Could you check a few things on this model? Use its own coordinates, in mm. A direction names the side the tool comes from. Give positions to 0.01 mm unless a question says otherwise; leave off trailing zeros. Loops run counter-clockwise (first coordinate to the right, second up) from the corner with the lowest first, then second, coordinate; pieces in that order, holes last. Notation, with made-up numbers: (29, 23) -> (55, 23) arc R30 cw to (55, 51) -> close; hole circle Ø4 at (68.25, -4.75). An arc over 180 degrees is marked (long way). Write item = value, one per line. Start each with the question number.
1) I want a section at A-A (z = 29). List the corners of the cut face in (x, y) for me.
2) On a 3-axis mill with a long thin cutter (end or side, diameter ignored), from which of +Z, -Z, +X, -X, +Y, -Y can I reach the whole of each face in a straight line? I mean faces 4 (the face through (2, -13.354, 20)), 5 (the face through (-5, 21.646, 19)), 6 (the face through (3.753, 26.484, 2.028)), 7 (the face through (5, -7.354, 20)). Say none if no direction works.
3) I'm going to push flat-ended pins straight in: pin 1 Ø10 at (x, z) = (-2, 14.5) entering from -Y; pin 2 Ø1.5 at (x, y) = (7, -14) entering from -Z; pin 3 Ø3.5 at (x, z) = (4.87, 22) entering from +Y; pin 4 Ø2 at (x, z) = (-5.5, 16) entering from +Y. Where does each tip first touch, or does it pass through?
4) If we mould it in two halves opening along Z, with no side actions, what happens to faces 1 (the face through (4.674, -10.396, 23.487)), 2 (the face through (2, -24, 4)), 3 (the face through (-2.631, 7, 19))? For each: +Z half, -Z half, draft (parallel to the pull), parting line (faces both ways), or undercut.
5) I want a section at D-D (x = 2.25). List the corners of the cut face in (y, z) for me, and give its area (3 significant figures).
6) I want a section at B-B (x = 7.75). List the corners of the cut face in (y, z) for me, and give its area (3 significant figures).
7) I need wall thicknesses on probe 1 along Y at (x, z) = (3.5, 6); probe 2 along X at (y, z) = (14.5, 28.5); probe 3 along Z at (x, y) = (9.75, 12.5). Which ranges of each line are inside material? Lowest first, please. Write a range as from..to.
8) I want a section at C-C (y = 5.5). List the corners of the cut face in (x, z) for me, and give its area (3 significant figures).
from build123d import *

# Parameters (mm, degrees)
BOSS_EXTRUDE1_DEPTH = 35
SKETCH3_R           = 1.5
CUT_EXTRUDE1_DEPTH  = 15
LPATTERN1_COUNT     = 3
LPATTERN1_PITCH     = 7
SKETCH6_W           = 15
SKETCH6_H           = 35
SKETCH6_R           = 1.5
BOSS_EXTRUDE4_DEPTH = 6
SKETCH7_W           = 15
SKETCH7_H           = 35
CUT_EXTRUDE2_DEPTH  = 8
SKETCH2_W           = 4
SKETCH2_H           = 35
BOSS_EXTRUDE5_DEPTH = 20
BOSS_EXTRUDE6_DEPTH = 15
SKETCH10_W          = 20
SKETCH10_H          = 4
BOSS_EXTRUDE7_DEPTH = 15
SKETCH11_R          = 3
CUT_EXTRUDE3_DEPTH  = 15


with BuildPart() as part:
    # Sketch1 → Boss-Extrude1 (new body)
    with BuildSketch(Plane.XY):
        Polygon((12.368951074, 15.64566438), (-2.631048926, 15.64566438), (-2.631048926, -13.35433562), (-7.631048926, -13.35433562), (-7.631048926, 21.64566438), (12.368951074, 21.64566438), align=None)
    extrude(amount=BOSS_EXTRUDE1_DEPTH)

    # Sketch3 → Cut-Extrude1 (cut)
    with BuildSketch(Plane.XZ.offset(-15.64566438)):
        with Locations((4.868951074, 29)):
            Circle(SKETCH3_R)
    cut_extrude1 = extrude(amount=-CUT_EXTRUDE1_DEPTH, mode=Mode.SUBTRACT)

    # LPattern1: Cut-Extrude1 ×3
    with Locations(*[(0, 0, -i * LPATTERN1_PITCH) for i in range(1, LPATTERN1_COUNT)]):
        add(cut_extrude1, mode=Mode.SUBTRACT)

    # Sketch6 → Boss-Extrude4 (add)
    with BuildSketch(Plane.XZ.offset(13.35433562)):
        with Locations((4.868951074, 17.5)):
            Rectangle(SKETCH6_W, SKETCH6_H)
        with Locations((4.868951074, 15)):
            Circle(SKETCH6_R, mode=Mode.SUBTRACT)
        with Locations((4.868951074, 29)):
            Circle(SKETCH6_R, mode=Mode.SUBTRACT)
        with Locations((4.868951074, 22)):
            Circle(SKETCH6_R, mode=Mode.SUBTRACT)
    extrude(amount=-BOSS_EXTRUDE4_DEPTH)

    # Sketch7 → Cut-Extrude2 (cut)
    with BuildSketch(Plane.XZ.offset(-15.64566438)):
        with Locations((4.868951074, 17.5)):
            Rectangle(SKETCH7_W, SKETCH7_H)
    extrude(amount=-CUT_EXTRUDE2_DEPTH, mode=Mode.SUBTRACT)

    # Sketch2 → Boss-Extrude5 (add)
    with BuildSketch(Plane.ZY.offset(7.631048926)):
        with Locations((2, 4.14566438)):
            Rectangle(SKETCH2_W, SKETCH2_H)
    extrude(amount=-BOSS_EXTRUDE5_DEPTH)

    # Sketch9 → Boss-Extrude6 (add)
    with BuildSketch(Plane(origin=(0, 21.64566438, 0), x_dir=(1, 0, 0), z_dir=(0, 1, 0))):
        Polygon((-2.631048926, -4), (-7.631048926, -4), (-7.631048926, 0), (12.368951074, 0), (12.368951074, -4), align=None)
    extrude(amount=BOSS_EXTRUDE6_DEPTH)

    # Sketch10 → Boss-Extrude7 (add)
    with BuildSketch(Plane.XZ.offset(13.35433562)):
        with Locations((2.368951074, 2)):
            Rectangle(SKETCH10_W, SKETCH10_H)
    extrude(amount=BOSS_EXTRUDE7_DEPTH)

    # Sketch11 → Cut-Extrude3 (cut)
    with BuildSketch(Plane.XY.offset(4)):
        with Locations((2.368951074, -20.85433562)):
            Circle(SKETCH11_R)
        with Locations((2.368951074, 29.14566438)):
            Circle(SKETCH11_R)
    extrude(amount=-CUT_EXTRUDE3_DEPTH, mode=Mode.SUBTRACT)


solid = part.part
Answer list:
q1.outline = (-7.63, -13.35) -> (3.37, -13.35) -> (3.37, -7.35) -> (-2.63, -7.35) -> (-2.63, 21.65) -> (-7.63, 21.65) -> close; (6.37, -13.35) -> (12.37, -13.35) -> (12.37, -7.35) -> (6.37, -7.35) -> close
q2.face_4 = +Z, +X, -X, -Y
q2.face_5 = +Z, +X, -X, +Y
q2.face_6 = +Z, -Z
q2.face_7 = +Z, +X, +Y
q3.pin_1 = -13.35
q3.pin_2 = 0
q3.pin_3 = -7.35
q3.pin_4 = 21.65
q4.face_1 = undercut
q4.face_2 = +Z half
q4.face_3 = draft
q5.outline = (-28.35, 0) -> (-23.85, 0) -> (-23.85, 4) -> (-28.35, 4) -> close; (-17.86, 0) -> (26.15, 0) -> (26.15, 4) -> (-7.35, 4) -> (-7.35, 35) -> (-13.35, 35) -> (-13.35, 4) -> (-17.86, 4) -> close; (32.14, 0) -> (36.65, 0) -> (36.65, 4) -> (32.14, 4) -> close
q5.area = 398 mm^2
q6.outline = (-28.35, 0) -> (36.65, 0) -> (36.65, 4) -> (-7.35, 4) -> (-7.35, 35) -> (-13.35, 35) -> (-13.35, 4) -> (-28.35, 4) -> close
q6.area = 446 mm^2
q7.probe_1 = -13.35..-7.35
q7.probe_2 = -7.63..-2.63
q7.probe_3 = 0..4
q8.outline = (-7.63, 0) -> (12.37, 0) -> (12.37, 4) -> (-2.63, 4) -> (-2.63, 35) -> (-7.63, 35) -> close
q8.area = 235 mm^2
